Geometry check sheet. Reference: the model listing, model coordinates, mm. A direction names the side the tool comes from. Round coordinates to 2 decimals unless told otherwise and drop trailing zeros. Write each loop counter-clockwise with the first axis right and the second up, starting at its lowest first coordinate (ties: lowest second). Pieces come first, ordered by that corner, then holes. Notation, with made-up numbers: (3.25, -39.5) -> (43.25, -39.5) arc R21 cw to (43.25, -19.5) -> close; hole circle Ø4 at (21.25, 50.25). An arc over 180 degrees is marked (long way). One line per question, with ' | ' between items.
```python
from build123d import *

# Parameters (mm, degrees)
SKETCH2_W           = 42
SKETCH2_H           = 42
BOSS_EXTRUDE1_DEPTH = 28
SKETCH3_R           = 1.5
CUT_EXTRUDE1_DEPTH  = 10
SKETCH4_R           = 12
BOSS_EXTRUDE2_DEPTH = 2
SKETCH5_R           = 10
CUT_EXTRUDE2_DEPTH  = 2
SKETCH6_R           = 2.5
BOSS_EXTRUDE3_DEPTH = 20
SKETCH7_W           = 15
SKETCH7_H           = 8
BOSS_EXTRUDE4_DEPTH = 6
SKETCH8_W           = 13
SKETCH8_H           = 6
CUT_EXTRUDE4_DEPTH  = 6


with BuildPart() as part:
    # Sketch2 → Boss-Extrude1 (new body)
    with BuildSketch(Plane.XY):
        Rectangle(SKETCH2_W, SKETCH2_H)
    extrude(amount=BOSS_EXTRUDE1_DEPTH)

    # Sketch3 → Cut-Extrude1 (cut)
    with BuildSketch(Plane.XY.offset(28)):
        with Locations((15.5, 15.5)):
            Circle(SKETCH3_R)
        with Locations((-15.5, 15.5)):
            Circle(SKETCH3_R)
        with Locations((-15.5, -15.5)):
            Circle(SKETCH3_R)
        with Locations((15.5, -15.5)):
            Circle(SKETCH3_R)
    extrude(amount=-CUT_EXTRUDE1_DEPTH, mode=Mode.SUBTRACT)

    # Sketch4 → Boss-Extrude2 (add)
    with BuildSketch(Plane.XY.offset(28)):
        Circle(SKETCH4_R)
    extrude(amount=BOSS_EXTRUDE2_DEPTH)

    # Sketch5 → Cut-Extrude2 (cut)
    with BuildSketch(Plane.XY.offset(30)):
        Circle(SKETCH5_R)
    extrude(amount=-CUT_EXTRUDE2_DEPTH, mode=Mode.SUBTRACT)

    # Sketch6 → Boss-Extrude3 (add)
    with BuildSketch(Plane.XY.offset(28)):
        Circle(SKETCH6_R)
    extrude(amount=BOSS_EXTRUDE3_DEPTH)

    # Sketch7 → Boss-Extrude4 (add)
    with BuildSketch(Plane.XZ.offset(21)):
        with Locations((0, 4)):
            Rectangle(SKETCH7_W, SKETCH7_H)
    extrude(amount=BOSS_EXTRUDE4_DEPTH)

    # Sketch8 → Cut-Extrude4 (cut)
    with BuildSketch(Plane(origin=(0, -27, 0), x_dir=(-1, 0, 0), z_dir=(0, -1, 0))):
        with Locations((0, -4)):
            Rectangle(SKETCH8_W, SKETCH8_H)
    extrude(amount=-CUT_EXTRUDE4_DEPTH, mode=Mode.SUBTRACT)


solid = part.part
```
(1) Go/stop test with flat-tipped pins: pin 1 (6.5 mm diameter, centred on x = 2, y = -24.5, fed in from +Z); pin 2 (10 mm diameter, centred on x = -14, z = 30, fed in from -Y); pin 3 (3 mm diameter, centred on y = -23, z = 4, fed in from +X); pin 4 (1.5 mm diameter, centred on x = -14.5, z = 30.5, fed in from +Y). Record where each tip stops, or that it passes through.
Resolved:
pin 1: stops at z = 8 | pin 2: stops at y = -21 | pin 3: stops at x = 7.5 | pin 4: passes through
(2) Sectioned sample at D-D on z = 16. Record the cut outline in (x, y), then the cut area to 3 significant figures.
Resolved:
outline: (-21, -21) -> (21, -21) -> (21, 21) -> (-21, 21) -> close | area: 1,760 mm2
(3) Sectioned sample at C-C on y = -15.5. Record the cut outline in (x, z), then the cut area to 3 significant figures.
Resolved:
outline: (-21, 0) -> (21, 0) -> (21, 28) -> (17, 28) -> (17, 18) -> (14, 18) -> (14, 28) -> (-14, 28) -> (-14, 18) -> (-17, 18) -> (-17, 28) -> (-21, 28) -> close | area: 1,120 mm2
(4) Sectioned sample at A-A on y = -23. Record the cut outline in (x, z), then the cut area to 3 significant figures.
Resolved:
outline: (-7.5, 0) -> (7.5, 0) -> (7.5, 8) -> (-7.5, 8) -> close; hole (-6.5, 1) -> (6.5, 1) -> (6.5, 7) -> (-6.5, 7) -> close | area: 42.0 mm2
(5) Material ranges on line 1 (Y direction, x = 0, z = 28.95); line 2 (Y direction, x = -15.5, z = 23.75); line 3 (Z direction, x = -9, y = 11), recorded low to high.
Resolved:
line 1: y = -12 to -10, -2.5 to 2.5, 10 to 12 | line 2: y = -21 to -17, -14 to 14, 17 to 21 | line 3: z = 0 to 28
(6) Draft check along X on faces 1 (the flat face through (-21, 0, 14)), 2 (the flat face through (-5, 9, 30)), 3 (the flat face through (0, -24, 7)), 4 (the flat face through (-6.5, -24, 4)). Enter one of: +X half, -X half, draft (parallel to the pull), parting line (faces both ways), or undercut.
Resolved:
face 1: -X half | face 2: draft | face 3: undercut | face 4: undercut
(7) Sectioned sample at B-B on x = 0. Record the cut outline in (y, z).
Resolved:
outline: (-27, 0) -> (21, 0) -> (21, 28) -> (12, 28) -> (12, 30) -> (10, 30) -> (10, 28) -> (2.5, 28) -> (2.5, 48) -> (-2.5, 48) -> (-2.5, 28) -> (-10, 28) -> (-10, 30) -> (-12, 30) -> (-12, 28) -> (-21, 28) -> (-21, 8) -> (-27, 8) -> (-27, 7) -> (-21, 7) -> (-21, 1) -> (-27, 1) -> close
(8) Access from +Z, -Z, +X, -X, +Y, -Y to the whole of each face (thin tool, end or side, straight path). Record for faces 5 (the flat face through (0, -21, 4)), 6 (the flat face through (-7.5, -24, 4)), 7 (the flat face through (0, -24, 8)), 8 (the cylindrical face through (14, -15.43, 23.07)), 9 (the flat face through (0, 21, 14)).
Resolved:
face 5: -Y | face 6: +Z, -Z, -X, -Y | face 7: +Z, +X, -X, -Y | face 8: +Z | face 9: +Z, -Z, +X, -X, +Y
